```python
from build123d import *

# Parameters (mm, degrees)
SKETCH_1_R         = 4.5
SKETCH_1_R_2       = 2.5
EXTRUDE_1_DEPTH    = 6.5
SKETCH_2_R         = 3.5
EXTRUDE_2_DEPTH    = 7
SKETCH_3_R         = 4.5
SKETCH_3_R_2       = 2.5
EXTRUDE_3_DEPTH    = 6.5
CHAMFER_1_SIZE2    = 1
CHAMFER_1_SIZE     = 0.5
CHAMFER_2_SIZE2    = 0.5
CHAMFER_2_SIZE     = 1
HOLE_WIZARD_M3_1_D = 2.5
HOLE_WIZARD_M3_2_D = 2.5


with BuildPart() as part:
    # 草图1 → 凸台-拉伸1 (new body)
    with BuildSketch(Plane(origin=(0, 0, 0), x_dir=(1, 0, 0), z_dir=(0, 1, 0))):
        with Locations(Location((0, 0, 0), (0, 0, 90))):
            Circle(SKETCH_1_R)
        with Locations(Location((0, 0, 0), (0, 0, 90))):
            Circle(SKETCH_1_R_2, mode=Mode.SUBTRACT)
    extrude(amount=EXTRUDE_1_DEPTH)

    # 草图2 → 凸台-拉伸2 (add)
    with BuildSketch(Plane(origin=(0, 6.5, 0), x_dir=(1, 0, 0), z_dir=(0, 1, 0))):
        with Locations(Location((0, 0, 0), (0, 0, 270))):
            Circle(SKETCH_2_R)
    extrude(amount=EXTRUDE_2_DEPTH)

    # 草图3 → 凸台-拉伸3 (add)
    with BuildSketch(Plane(origin=(0, 13.5, 0), x_dir=(1, 0, 0), z_dir=(0, 1, 0))):
        with Locations(Location((0, 0, 0), (0, 0, 90))):
            Circle(SKETCH_3_R)
        with Locations(Location((0, 0, 0), (0, 0, 90))):
            Circle(SKETCH_3_R_2, mode=Mode.SUBTRACT)
    extrude(amount=EXTRUDE_3_DEPTH)

    # 倒角1
    chamfer_1_edges = [part.edges().sort_by_distance(p)[0] for p in [
        (0, 6.5, 4.5),
    ]]
    chamfer_1_side = [part.faces().sort_by_distance(p)[0] for p in [
        (0, 6.49, 4.5),
    ]]
    chamfer(chamfer_1_edges, length=CHAMFER_1_SIZE - 0.0001, length2=CHAMFER_1_SIZE2 - 0.0001, reference=chamfer_1_side[0])  # a hair under: the kernel refuses the full size

    # 倒角2
    chamfer_2_edges = [part.edges().sort_by_distance(p)[0] for p in [
        (0, 13.5, 4.5),
    ]]
    chamfer_2_side = [part.faces().sort_by_distance(p)[0] for p in [
        (0, 13.5, 4.49),
    ]]
    chamfer(chamfer_2_edges, length=CHAMFER_2_SIZE - 0.0001, length2=CHAMFER_2_SIZE2 - 0.0001, reference=chamfer_2_side[0])  # a hair under: the kernel refuses the full size

    # M3 螺纹孔1 (through all)
    with Locations(Plane(origin=(4.499987687, 2.904707671, -0.01052714), x_dir=(0.002339364434, 0, 0.999997263683), z_dir=(0.999997263683, 0, -0.002339364434))):
        with Locations((0, 0)):
            Hole(HOLE_WIZARD_M3_1_D / 2)

    # M3 螺纹孔2 (through all)
    with Locations(Plane(origin=(4.499987687, 17.116346609, -0.01052714), x_dir=(0.002339364434, 0, 0.999997263683), z_dir=(0.999997263683, 0, -0.002339364434))):
        with Locations((0, 0)):
            Hole(HOLE_WIZARD_M3_2_D / 2)


solid = part.part
```
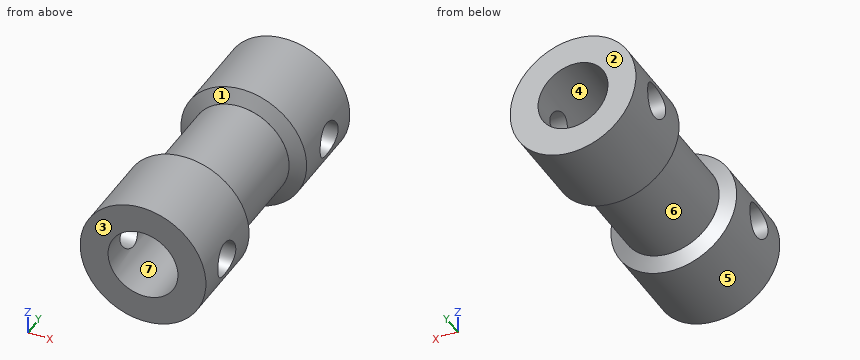
Check sheet for the modelled part. Datum: model origin and axes. Units: mm. Face numbers are marked on the shaded views. A direction names the side the tool comes from. Coordinates: 2 decimals unless noted, no trailing zeros. Write each loop counter-clockwise with the first axis right and the second up, starting at its lowest first coordinate (ties: lowest second). Pieces come first, ordered by that corner, then holes. Notation, with made-up numbers: M 71.5,48.5 L 91.5,48.5 A19 ccw 91.5,85.5 Z; hole C 12.5,-11.5 d11. An arc over 180 degrees is marked long. Use one line per item in the form item = value.
Item 1: Material ranges on L1, parallel to X at y = 5, z = 0; L2, parallel to Y at x = 3, z = 0.25; L3, parallel to X at y = 10.5, z = 0, recorded low to high. Write a range as from..to.
Answer below:
L1 = -4.5..-2.5, 2.5..4.5
L2 = 0..1.68, 4.13..15.89, 18.34..20
L3 = -3.5..3.5
Item 2: Sectioned sample at C-C, the plane x = 3.75. State how many separate pieces and enclosed holes the cut face has, and give its area (3 significant figures).
Answer below:
separate_pieces = 2
enclosed_holes = 2
area = 52.3 mm^2
Item 3: Gauge pin test, flat ends, axial feed: pin 1 Ø3 at (x, z) = (0, 0) entering from -Y; pin 2 Ø2 at (y, z) = (17, -2.5) entering from +X. Record the tip position at first contact, or that the pin passes through.
Answer below:
pin_1 = 6.5
pin_2 = 4.24
Item 4: Set-up check for the marked faces 4, 5, 6 and 7: record each of +Z, -Z, +X, -X, +Y, -Y from which the full face is reachable in a straight line by a thin tool's end or side.
Answer below:
face_4 = +Y
face_5 = +Y, -Y
face_6 = none
face_7 = -Y
Item 5: Sectioned sample at A-A, the plane y = 3.25. Record the cut outline in (x, z).
Answer below:
outline = M -4.34,-1.19 A4.5 ccw 4.33,-1.21 L 2.19,-1.21 A2.5 cw -2.2,-1.2 Z; M -4.33,1.21 L -2.19,1.21 A2.5 cw 2.2,1.2 L 4.34,1.19 A4.5 ccw Z
Item 6: Release check for a two-part mould opening along Y. For the marked faces 1, 2 and 3 record: pulls with the +Y half, pulls with the -Y half, needs draft (parallel to the pull), parting line crosses it, or undercut.
Answer below:
face_1 = undercut
face_2 = pulls with the +Y half
face_3 = pulls with the -Y half
